The model under review builds one solid part; all positions refer to its coordinate system, in mm. Face numbers are marked on the shaded views. A direction names the side the tool comes from. Give positions to 0.01 mm unless a question says otherwise; leave off trailing zeros. Loops run counter-clockwise (first coordinate to the right, second up) from the corner with the lowest first, then second, coordinate; pieces in that order, holes last. Notation, with made-up numbers: M 84,89.5 L 98,89.5 A20 ccw 98,119.5 Z; hole C -13,42 d9. An arc over 180 degrees is marked long. Write item = value, one per line. Start each with the question number.
1. For the marked faces 4, 5, 6, 7 and 8, list the 3-axis set-ups (+Z, -Z, +X, -X, +Y, -Y) from which the entire face can be reached by the end or side of a thin tool; tool diameter is ignored.
2. We need section B-B on y = 0. Give the boundary of the cut face in (x, z).
3. We need section C-C on y = -15. Give the boundary of the cut face in (x, z).
4. Draft analysis for pull direction Y (two halves, no side actions). For the marked faces 1, 2 and 3, state which applies: pulls with the +Y half, pulls with the -Y half, needs draft (parallel to the pull), parting line crosses it, or undercut.
5. We need section A-A on x = 0. Give the boundary of the cut face in (y, z), then the cut area to 3 significant figures.
6. For pin 1 (4 mm diameter, centred on y = 1.5, z = 0, fed in from +X); pin 2 (3 mm diameter, centred on y = 17.5, z = 0, fed in from -X); pin 3 (1 mm diameter, centred on y = -9, z = 2.5, fed in from -X); pin 4 (1.5 mm diameter, centred on x = 6.5, y = -6.5, fed in from -Z) (3 decimals), all flat-tipped, find the tip position at first contact; note any pin that passes through.
7. Wall thickness on line 1 along Y through (x, z) = (0, 1.25); line 2 along X through (y, z) = (-5, 0.5); line 3 along Y through (x, z) = (-5.5, -0.5): over which ranges is each line inside the solid? List them lowest first. Write a range as from..to.
8. We need section D-D on x = 13. Give the boundary of the cut face in (y, z), then the cut area to 3 significant figures.
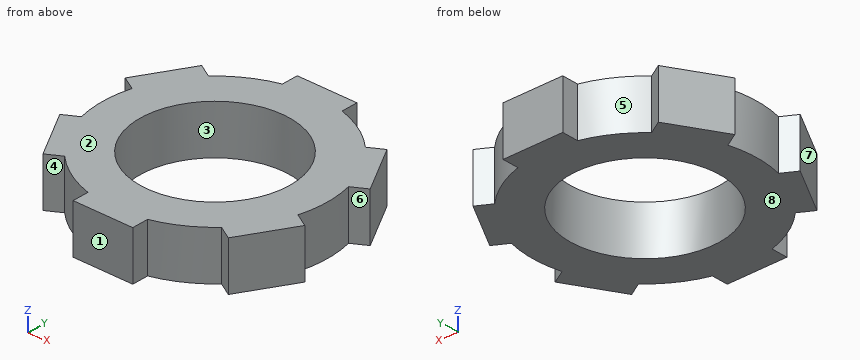
from build123d import *

# Parameters (mm, degrees)
SKETCH2_R           = 17.25
SKETCH2_R_2         = 11.5
BOSS_EXTRUDE1_DEPTH = 3.75
BOSS_EXTRUDE2_START = -3.75
SKETCH3_W           = 9.2
SKETCH3_H           = 2.53
BOSS_EXTRUDE2_DEPTH = 7.5
CIRPATTERN1_COUNT   = 6


with BuildPart() as part:
    # Sketch2 → Boss-Extrude1 (new body, symmetric)
    with BuildSketch(Plane.XY):
        Circle(SKETCH2_R)
        Circle(SKETCH2_R_2, mode=Mode.SUBTRACT)
    extrude(amount=BOSS_EXTRUDE1_DEPTH, both=True)

    # Sketch3 → Boss-Extrude2 (add)
    with BuildSketch(Plane.XY.offset(BOSS_EXTRUDE2_START)):
        with Locations((0, 17.894)):
            Rectangle(SKETCH3_W, SKETCH3_H)
    boss_extrude2 = extrude(amount=BOSS_EXTRUDE2_DEPTH)

    # CirPattern1: Boss-Extrude2 ×6 about axis
    cirpattern1_axis = Axis((0, 0, 0), (0, 0, 1))
    for i in range(1, CIRPATTERN1_COUNT):
        add(boss_extrude2.rotate(cirpattern1_axis, i * 360 / CIRPATTERN1_COUNT))


solid = part.part
Final values:
q1.face_4 = +Z, -Z, -Y
q1.face_5 = +Z, -Z, +Y
q1.face_6 = +Z, -Z, +X
q1.face_7 = +Z, -Z, -X, -Y
q1.face_8 = -Z, +X, -X, +Y, -Y
q2.outline = M -17.25,-3.75 L -11.5,-3.75 L -11.5,3.75 L -17.25,3.75 Z; M 11.5,-3.75 L 17.25,-3.75 L 17.25,3.75 L 11.5,3.75 Z
q3.outline = M -8.52,-3.75 L 8.52,-3.75 L 8.52,3.75 L -8.52,3.75 Z
q4.face_1 = pulls with the -Y half
q4.face_2 = needs draft
q4.face_3 = undercut
q5.outline = M -19.16,-3.75 L -11.5,-3.75 L -11.5,3.75 L -19.16,3.75 Z; M 11.5,-3.75 L 19.16,-3.75 L 19.16,3.75 L 11.5,3.75 Z
q5.area = 115 mm²
q6.pin_1 = 17.25
q6.pin_2 = -6.45
q6.pin_3 = -17.22
q6.pin_4 = through
q7.line_1 = -19.16..-11.5, 11.5..19.16
q7.line_2 = -17.86..-10.36, 10.36..17.86
q7.line_3 = -16.35..-10.1, 10.1..16.35
q8.outline = M -12.82,-3.75 L 12.82,-3.75 L 12.82,3.75 L -12.82,3.75 Z
q8.area = 192 mm²
